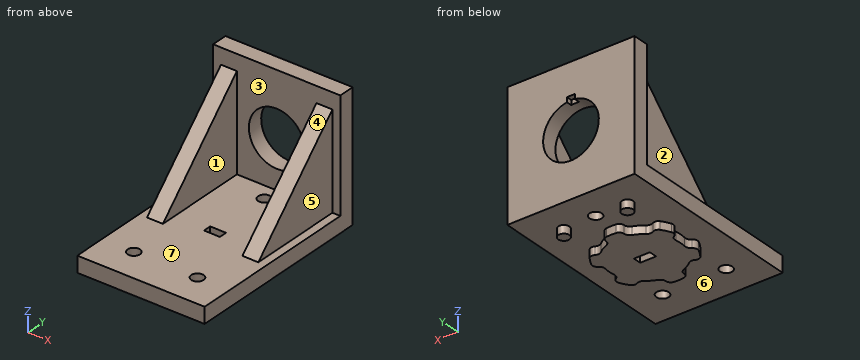
```python
from build123d import *

# Parameters (mm, degrees)
SKETCH1_W           = 50.8
SKETCH1_H           = 76.2
SKETCH1_R           = 2.4765
BOSS_EXTRUDE1_DEPTH = 6.35
SKETCH2_R           = 2.2225
BOSS_EXTRUDE2_DEPTH = 3.175
SKETCH3_W           = 6.35
SKETCH3_H           = 3.175
CUT_EXTRUDE1_DEPTH  = 10.525
SKETCH4_W           = 50.8
SKETCH4_H           = 44.45
BOSS_EXTRUDE3_DEPTH = 6.35
BOSS_EXTRUDE4_DEPTH = 22.225
SKETCH6_W           = 31.75
SKETCH6_H           = 38.1
CUT_EXTRUDE2_DEPTH  = 45.45
SKETCH7_R           = 11.1125
CUT_EXTRUDE3_DEPTH  = 7.35
SKETCH8_W           = 3.175
SKETCH8_H           = 1.905
CUT_EXTRUDE4_DEPTH  = 2.2225


with BuildPart() as part:
    # Sketch1 → Boss-Extrude1 (new body)
    with BuildSketch(Plane.XY):
        Rectangle(SKETCH1_W, SKETCH1_H)
        with Locations((-12.7, -25.4)):
            Circle(SKETCH1_R, mode=Mode.SUBTRACT)
        with Locations((12.7, -25.4)):
            Circle(SKETCH1_R, mode=Mode.SUBTRACT)
        with Locations((0, 25.4)):
            Circle(SKETCH1_R, mode=Mode.SUBTRACT)
    extrude(amount=BOSS_EXTRUDE1_DEPTH)

    # Sketch2 → Boss-Extrude2 (add)
    with BuildSketch(Plane(origin=(0, 0, 0), x_dir=(-1, 0, 0), z_dir=(0, 0, -1))):
        with Locations((-12.7, 25.4)):
            Circle(SKETCH2_R)
        with Locations((12.7, 25.4)):
            Circle(SKETCH2_R)
        with BuildLine():
            ThreePointArc((-5.08, 13.340296662), (-7.1374, 12.362339434), (-9.013035804, 11.069557382))
            ThreePointArc((-9.013035804, 11.069557382), (-10.265964814, 10.566776235), (-11.582919047, 10.863847829))
            ThreePointArc((-11.582919047, 10.863847829), (-12.926326796, 11.078530787), (-14.070368319, 10.342322835))
            ThreePointArc((-14.070368319, 10.342322835), (-15.122968614, 8.73125), (-15.991898469, 7.014134987))
            ThreePointArc((-15.991898469, 7.014134987), (-16.057452496, 5.65526199), (-15.199827727, 4.59917823))
            ThreePointArc((-15.199827727, 4.59917823), (-14.284079063, 3.607198205), (-14.093035804, 2.27073928))
            ThreePointArc((-14.093035804, 2.27073928), (-14.2748, 0), (-14.093035804, -2.27073928))
            ThreePointArc((-14.093035804, -2.27073928), (-14.284079063, -3.607198205), (-15.199827727, -4.59917823))
            ThreePointArc((-15.199827727, -4.59917823), (-16.057452496, -5.65526199), (-15.991898469, -7.014134987))
            ThreePointArc((-15.991898469, -7.014134987), (-15.122968614, -8.73125), (-14.070368319, -10.342322835))
            ThreePointArc((-14.070368319, -10.342322835), (-12.926326796, -11.078530787), (-11.582919047, -10.863847829))
            ThreePointArc((-11.582919047, -10.863847829), (-10.265964814, -10.566776235), (-9.013035804, -11.069557382))
            ThreePointArc((-9.013035804, -11.069557382), (-7.1374, -12.362339434), (-5.08, -13.340296662))
            ThreePointArc((-5.08, -13.340296662), (-4.018114249, -14.173974441), (-3.616908679, -15.46302606))
            ThreePointArc((-3.616908679, -15.46302606), (-3.1311257, -16.733792777), (-1.92153015, -17.356457822))
            ThreePointArc((-1.92153015, -17.356457822), (0, -17.4625), (1.92153015, -17.356457822))
            ThreePointArc((1.92153015, -17.356457822), (3.1311257, -16.733792777), (3.616908679, -15.46302606))
            ThreePointArc((3.616908679, -15.46302606), (4.018114249, -14.173974441), (5.08, -13.340296662))
            ThreePointArc((5.08, -13.340296662), (7.1374, -12.362339434), (9.013035804, -11.069557382))
            ThreePointArc((9.013035804, -11.069557382), (10.265964814, -10.566776235), (11.582919047, -10.863847829))
            ThreePointArc((11.582919047, -10.863847829), (12.926326796, -11.078530787), (14.070368319, -10.342322835))
            ThreePointArc((14.070368319, -10.342322835), (15.122968614, -8.73125), (15.991898469, -7.014134987))
            ThreePointArc((15.991898469, -7.014134987), (16.057452496, -5.65526199), (15.199827727, -4.59917823))
            ThreePointArc((15.199827727, -4.59917823), (14.284079063, -3.607198205), (14.093035804, -2.27073928))
            ThreePointArc((14.093035804, -2.27073928), (14.2748, 0), (14.093035804, 2.27073928))
            ThreePointArc((14.093035804, 2.27073928), (14.284079063, 3.607198205), (15.199827727, 4.59917823))
            ThreePointArc((15.199827727, 4.59917823), (16.057452496, 5.65526199), (15.991898469, 7.014134987))
            ThreePointArc((15.991898469, 7.014134987), (15.122968614, 8.73125), (14.070368319, 10.342322835))
            ThreePointArc((14.070368319, 10.342322835), (12.926326796, 11.078530787), (11.582919047, 10.863847829))
            ThreePointArc((11.582919047, 10.863847829), (10.265964814, 10.566776235), (9.013035804, 11.069557382))
            ThreePointArc((9.013035804, 11.069557382), (7.1374, 12.362339434), (5.08, 13.340296662))
            ThreePointArc((5.08, 13.340296662), (4.018114249, 14.173974441), (3.616908679, 15.46302606))
            ThreePointArc((3.616908679, 15.46302606), (3.1311257, 16.733792777), (1.92153015, 17.356457822))
            ThreePointArc((1.92153015, 17.356457822), (0, 17.4625), (-1.92153015, 17.356457822))
            ThreePointArc((-1.92153015, 17.356457822), (-3.1311257, 16.733792777), (-3.616908679, 15.46302606))
            ThreePointArc((-3.616908679, 15.46302606), (-4.018114249, 14.173974441), (-5.08, 13.340296662))
        make_face()
    extrude(amount=BOSS_EXTRUDE2_DEPTH)

    # Sketch3 → Cut-Extrude1 (cut, through all)
    with BuildSketch(Plane(origin=(0, 0, -3.175), x_dir=(-1, 0, 0), z_dir=(0, 0, -1))):
        Rectangle(SKETCH3_W, SKETCH3_H)
    extrude(amount=-CUT_EXTRUDE1_DEPTH, mode=Mode.SUBTRACT)

    # Sketch4 → Boss-Extrude3 (add)
    with BuildSketch(Plane(origin=(0, 38.1, 0), x_dir=(1, 0, 0), z_dir=(0, 1, 0))):
        with Locations((0, -28.575)):
            Rectangle(SKETCH4_W, SKETCH4_H)
    extrude(amount=-BOSS_EXTRUDE3_DEPTH)

    # Sketch5 → Boss-Extrude4 (add, symmetric)
    with BuildSketch(Plane(origin=(0, 0, 0), x_dir=(0, 0, -1), z_dir=(1, 0, 0))):
        Polygon((-44.45, 31.75), (-6.35, -6.35), (-6.35, 31.75), align=None)
    extrude(amount=BOSS_EXTRUDE4_DEPTH, both=True)

    # Sketch6 → Cut-Extrude2 (cut, through all)
    with BuildSketch(Plane.XY.offset(6.35)):
        with Locations((0, 12.7)):
            Rectangle(SKETCH6_W, SKETCH6_H)
    extrude(amount=CUT_EXTRUDE2_DEPTH, mode=Mode.SUBTRACT)

    # Sketch7 → Cut-Extrude3 (cut, through all)
    with BuildSketch(Plane.XZ.offset(-31.75)):
        with Locations((0, 25.4)):
            Circle(SKETCH7_R)
    extrude(amount=-CUT_EXTRUDE3_DEPTH, mode=Mode.SUBTRACT)

    # Sketch8 → Cut-Extrude4 (cut)
    with BuildSketch(Plane(origin=(0, 38.1, 0), x_dir=(1, 0, 0), z_dir=(0, 1, 0))):
        with Locations((0, -37.351022628)):
            Rectangle(SKETCH8_W, SKETCH8_H)
    extrude(amount=-CUT_EXTRUDE4_DEPTH, mode=Mode.SUBTRACT)


solid = part.part
```
The listing builds one solid part. Answer for the finished solid, in the listing's coordinates (mm). Face numbers are marked on the shaded views. A direction names the side the tool comes from. Give positions to 0.01 mm unless a question says otherwise; leave off trailing zeros. Order: outer loops, then holes, each group sorted by start corner. A loop starts at its lowest first (then second) coordinate and runs counter-clockwise, first axis right, second up.
1) Consider line 1 along X through (y, z) = (-0.5, 8) (3 decimals); line 2 along X through (y, z) = (36, 25); line 3 along Z through (x, y) = (-1, -23.5). Determine where each line is inside the solid, lowest interval first.
Reported:
line 1: x = -22.225 to -15.875, 15.875 to 22.225
line 2: x = -25.4 to -11.11, 11.11 to 25.4
line 3: z = 0 to 6.35
2) For the marked faces 5, 6 and 7, determine the directions among +Z, -Z, +X, -X, +Y, -Y from which every point of the face is accessible in a straight line to the end or side of a thin tool.
Reported:
face 5: +Z, +X, -Y
face 6: -Z
face 7: +Z, -Y
3) Find section C-C on z = 4.5. Write down the section's boundary in (x, y) (1 decimal).
Reported:
outline: (-25.4, -38.1) - (25.4, -38.1) - (25.4, 38.1) - (-25.4, 38.1) - close; hole circle Ø5 at (-12.7, -25.4); hole (-3.2, -1.6) - (3.2, -1.6) - (3.2, 1.6) - (-3.2, 1.6) - close; hole circle Ø5 at (0, 25.4); hole circle Ø5 at (12.7, -25.4)
4) Find section D-D on y = -25.4. Write down the section's boundary in (x, z).
Reported:
outline: (-25.4, 0) - (-15.18, 0) - (-15.18, 6.35) - (-25.4, 6.35) - close; (-10.22, 0) - (10.22, 0) - (10.22, 6.35) - (-10.22, 6.35) - close; (15.18, 0) - (25.4, 0) - (25.4, 6.35) - (15.18, 6.35) - close
5) Determine the mould class of the marked faces 1, 2, 3 and 4 for opening direction X: pulls with the +X half, pulls with the -X half, needs draft (parallel to the pull), parting line crosses it, or undercut.
Reported:
face 1: undercut
face 2: pulls with the -X half
face 3: undercut
face 4: needs draft
6) Given P1, Ø0.7, axis at x = -0.5, y = 37.5, coming from the -Z side; P2, Ø8, axis at x = -20, y = -1.5, coming from the +Z side; P3, Ø0.6, axis at x = 1, z = 37.5, coming from the +Y side, each flat-ended and moving along its own axis, determine where each tip first touches the part or whether it passes through.
Reported:
P1: stops at z = 0
P2: stops at z = 15.2
P3: stops at y = 35.88
